The model under review builds one solid part; all positions refer to its coordinate system, in mm. Face numbers are marked on the shaded views. A direction names the side the tool comes from. Round coordinates to 2 decimals unless told otherwise and drop trailing zeros. Loops run counter-clockwise (first coordinate to the right, second up) from the corner with the lowest first, then second, coordinate; pieces in that order, holes last. Notation, with made-up numbers: M 23,71 L 47,71 A22 cw 47,81 Z; hole C -7,3 d8. An arc over 180 degrees is marked long. Return JSON: item names as keys, results as strings. Group by question number.
Q1. Clearance check with flat-ended pins moving along their axes: pin 1 Ø2 at (x, z) = (-40.5, 10.5) entering from -Y; pin 2 Ø2 at (x, y) = (-7.5, -27.5) entering from -Z. State where each tip first meets the part, or that it passes through.
Q2. Consider section C-C (x = -32). State the section outline as (y, z) points, and give its area (3 significant figures).
Q3. Consider section B-B (x = -39). State the section outline as (y, z) points, and give its area (3 significant figures).
Q4. For the marked faces 1 and 2, list the 3-axis set-ups (+Z, -Z, +X, -X, +Y, -Y) from which the entire face can be reached by the end or side of a thin tool; tool diameter is ignored.
Q5. Consider section A-A (z = 10.25). State the section outline as (x, y) points, and give its area (3 significant figures).
Q6. To check wall thickness, follow line 1 along Y through (x, z) = (-43, 4); line 2 along X through (y, z) = (-71.5, 5.5); line 3 along Z through (x, y) = (-2, -14). State the ranges of each line that lie inside material, in increasing order.
Q7. Draft analysis for pull direction X (two halves, no side actions). For the marked faces 3, 4, 5 and 6, state which applies: pulls with the +X half, pulls with the -X half, needs draft (parallel to the pull), parting line crosses it, or undercut.
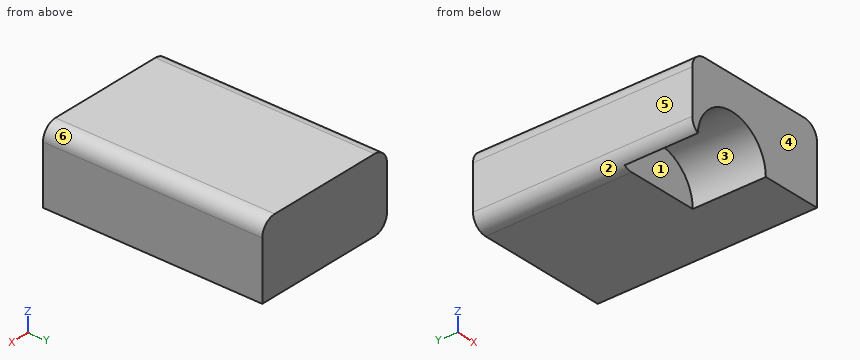
from build123d import *

# Parameters (mm, degrees)
F1_E0_TOP_W = 50.8
F1_E0_TOP_H = 25.4
F2_DEPTH    = 76.2
F3_R        = 5.08
F4_R        = 13.875567501
F5_DEPTH    = 25.4


with BuildPart() as f2:
    # F1_E0_top (on explicit) → F2 (new body)
    with BuildSketch(Plane(origin=(-50.8, 0, 0), x_dir=(1, 0, 0), z_dir=(0, -1, 0))):
        with Locations((25.4, 12.7)):
            Rectangle(F1_E0_TOP_W, F1_E0_TOP_H)
    extrude(amount=F2_DEPTH)

    # F3
    f3_edges = [f2.edges().sort_by_distance(p)[0] for p in [
        (-50.8, -38.1, 0),
        (-50.8, -38.1, 25.4),
        (0, -38.1, 25.4),
    ]]
    fillet(f3_edges, radius=F3_R)

    # F4 (on face) → F5 (cut)
    with BuildSketch(Plane.XZ.offset(76.2)):
        with Locations((-34.7172878683, 0)):
            Circle(F4_R)
    extrude(amount=-F5_DEPTH, mode=Mode.SUBTRACT)


solid = f2.part
Values:
{
 "1": {"pin 1": "stops at y = -50.8", "pin 2": "stops at z = 0"},
 "2": {"outline": "M -76.2,13.61 L -50.8,13.61 L -50.8,0 L 0,0 L 0,25.4 L -76.2,25.4 Z", "area": "1,590 mm2"},
 "3": {"outline": "M -76.2,13.2 L -50.8,13.2 L -50.8,0 L 0,0 L 0,25.4 L -76.2,25.4 Z", "area": "1,600 mm2"},
 "4": {"face 1": "-Z, -Y", "face 2": "-Z, -X, +Y, -Y"},
 "5": {"outline": "M -50.8,-76.2 L -44.07,-76.2 L -44.07,-50.8 L -25.36,-50.8 L -25.36,-76.2 L 0,-76.2 L 0,0 L -50.8,0 Z", "area": "3,400 mm2"},
 "6": {"line 1": "y = -50.8 to 0", "line 2": "x = -50.8 to -47.46, -21.98 to 0", "line 3": "z = 0 to 24.36"},
 "7": {"face 3": "undercut", "face 4": "needs draft", "face 5": "pulls with the -X half", "face 6": "pulls with the +X half"}
}
